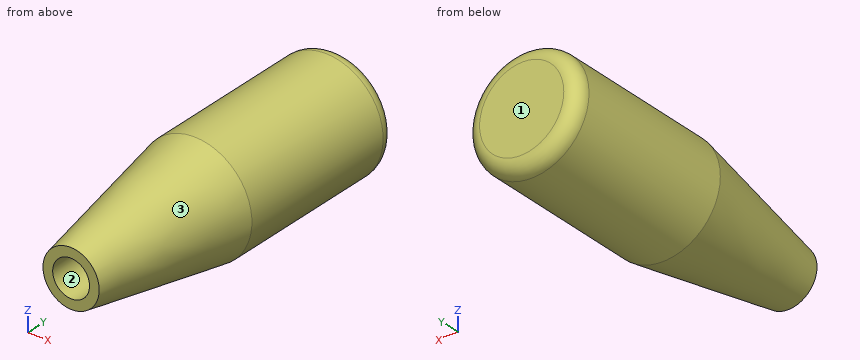
from build123d import *

# Parameters (mm, degrees)
F3_R     = 2
F5_D     = 5.25
F5_DEPTH = 14.8190481046


with BuildPart() as f2:
    # F0 (on Top) → F2 (revolve)
    with BuildSketch(Plane.XY):
        Polygon((0, -14.8180481046), (0, 32.7115394175), (-8, 32.7115394175), (-8, 7.3624262586), (-4.0073962882, -14.8180481046), align=None)
    revolve(axis=Axis((0, 8.853550069, 0), (0, -1, 0)))

    # F3
    f3_edges = [f2.edges().sort_by_distance(p)[0] for p in [
        (8, 32.711539, 0),
    ]]
    fillet(f3_edges, radius=F3_R)

    # F5 (through all, one way)
    with BuildSketch(Plane(origin=(0, 0, 0), x_dir=(1, 0, 0), z_dir=(0, 1, 0))):
        with Locations((0, 0)):
            Circle(F5_D / 2)
    extrude(amount=-F5_DEPTH, mode=Mode.SUBTRACT)


with BuildPart() as f2_1:
    # F6: moved
    add(f2.part.moved(Location((8, 0, 0))))


solid = f2_1.part
Work out the finished part from the listing and answer in its coordinate system (mm). Face numbers are marked on the shaded views. Round coordinates to 2 decimals unless told otherwise and drop trailing zeros. Loops run counter-clockwise (first coordinate to the right, second up) from the corner with the lowest first, then second, coordinate; pieces in that order, holes last. Notation, with made-up numbers: (-0.75, 76.5) -> (22.25, 76.5) arc R22 cw to (22.25, 92.5) -> close; hole circle Ø2 at (75.25, -27). An arc over 180 degrees is marked (long way). Use one line per item in the form item = value.
(1) Find section D-D on y = -9.5. Give the vertices of the cut face in (x, z) (3 decimals), then the cut area to 3 significant figures.
Answer list:
outline = circle Ø9.929 at (8, 0); hole circle Ø5.25 at (8, 0)
area = 55.8 mm2
(2) Find section A-A on z = 0. Give the vertices of the cut face in (x, y) (3 decimals).
Answer list:
outline = (0, 7.362) -> (3.993, -14.818) -> (5.375, -14.818) -> (5.375, 0) -> (10.625, 0) -> (10.625, -14.818) -> (12.007, -14.818) -> (16, 7.362) -> (16, 30.712) arc R2 ccw to (14, 32.712) -> (2, 32.712) arc R2 ccw to (0, 30.712) -> close
(3) Straight lines are drawn through the part: line 1 (Y direction, x = 9, z = 1.5); line 2 (Z direction, x = 8, y = -4.25) (3 decimals); line 3 (Z direction, x = 8, y = -11.25) (3 decimals). For each, find the intervals that lie inside material, in ascending order.
Answer list:
line_1 = 0 to 32.71
line_2 = -5.91 to -2.625, 2.625 to 5.91
line_3 = -4.65 to -2.625, 2.625 to 4.65
(4) For a pull along X with two mould halves and no side action, classify the marked faces 1, 2 and 3 as released by +X, released by -X, zero draft, split by the parting line, or undercut.
Answer list:
face_1 = zero draft
face_2 = undercut
face_3 = split by the parting line
(5) Find section B-B on x = 8. Give the vertices of the cut face in (y, z) (3 decimals).
Answer list:
outline = (-14.818, -4.007) -> (7.362, -8) -> (30.712, -8) arc R2 ccw to (32.712, -6) -> (32.712, 6) arc R2 ccw to (30.712, 8) -> (7.362, 8) -> (-14.818, 4.007) -> (-14.818, 2.625) -> (0, 2.625) -> (0, -2.625) -> (-14.818, -2.625) -> close
(6) Find section C-C on y = 8. Give the vertices of the cut face in (x, z), then the cut area to 3 significant figures.
Answer list:
outline = circle Ø16 at (8, 0)
area = 201 mm2
(7) Flat-ended cylindrical pins translate along their axes: P1, Ø4, axis at x = 12, y = 9, coming from the +Z side; P2, Ø1.6, axis at x = 9, z = 0.5, coming from the -Y side; P3, Ø1, axis at y = 5.5, z = -2, coming from the -X side. Find the tip coordinate at first contact, or state that the pin passes through.
Answer list:
P1 = 7.75
P2 = 0
P3 = 0.45
